Geometry check sheet. Reference: the model listing, model coordinates, mm. Face numbers are marked on the shaded views. A direction names the side the tool comes from. Coordinates: 2 decimals unless noted, no trailing zeros. Order: outer loops, then holes, each group sorted by start corner. A loop starts at its lowest first (then second) coordinate and runs counter-clockwise, first axis right, second up. Notation, with made-up numbers: M 79.25,8 L 93.25,8 A4 cw 93.25,14 Z; hole C 62.5,66 d6. An arc over 180 degrees is marked long. One line per item, written item: value. Start each with the question number.
1) Draft check along X on the marked faces 1, 2 and 3. Enter one of: pulls with the +X half, pulls with the -X half, needs draft (parallel to the pull), parting line crosses it, or undercut.
2) Sectioned sample at A-A, the plane x = 0. Enter the section's corners in (y, z), then the cut area to 3 significant figures.
3) Access from +Z, -Z, +X, -X, +Y, -Y to the whole of each face (thin tool, end or side, straight path). Record for the marked faces 4, 5 and 6.
4) Go/stop test with flat-tipped pins: P1, Ø2, axis at x = -2.5, z = -2, coming from the -Y side; P2, Ø1, axis at x = 0, z = 1, coming from the -Y side; P3, Ø0.5, axis at x = 0, z = -1, coming from the +Y side. Record where each tip stops, or that it passes through.
5) Thickness scan on L1, parallel to Z at x = -3.5, y = -3.5; L2, parallel to X at y = -1, z = -0.8; L3, parallel to Y at x = 0.25, z = -1.65. Record the ranges inside material, lowest first. Write a range as from..to.
```python
from build123d import *

# Parameters (mm, degrees)
SKETCH2_R           = 4.5
BOSS_EXTRUDE1_DEPTH = 3
CUT_EXTRUDE1_DEPTH  = 11.464224768
FILLET1_R           = 0.25


with BuildPart() as part:
    # Sketch1 → Revolve1 (revolve)
    with BuildSketch(Plane(origin=(0, 0, 0), x_dir=(1, 0, 0), z_dir=(0, 1, 0))):
        Polygon((6.5, 0), (0, 0), (0, -2), (6.395184442, -2), align=None)
    revolve(axis=Axis((0, 0, 0), (0, 0, 1)))

    # Sketch2 → Boss-Extrude1 (add)
    with BuildSketch(Plane(origin=(0, 0, 0), x_dir=(-1, 0, 0), z_dir=(0, 0, -1))):
        with Locations(Location((0, 0, 0), (0, 0, 90))):
            Circle(SKETCH2_R)
    extrude(amount=BOSS_EXTRUDE1_DEPTH)

    # Sketch3 → Cut-Extrude1 (cut, through all)
    with BuildSketch(Plane.XY.offset(2)):
        with BuildLine():
            Line((1.568375673, 2.283493649), (1.443375673, 2.5))
            Line((1.443375673, 2.5), (1.193375673, 2.5))
            ThreePointArc((1.193375673, 2.5), (1.043375673, 2.445), (0.893375673, 2.5))
            Line((0.893375673, 2.5), (-0.893375673, 2.5))
            ThreePointArc((-0.893375673, 2.5), (-1.043375673, 2.445), (-1.193375673, 2.5))
            Line((-1.193375673, 2.5), (-1.443375673, 2.5))
            Line((-1.443375673, 2.5), (-1.568375673, 2.283493649))
            ThreePointArc((-1.568375673, 2.283493649), (-1.595744276, 2.126089838), (-1.718375673, 2.023686028))
            Line((-1.718375673, 2.023686028), (-2.611751346, 0.476313972))
            ThreePointArc((-2.611751346, 0.476313972), (-2.639119949, 0.318910162), (-2.761751346, 0.216506351))
            Line((-2.761751346, 0.216506351), (-2.886751346, 0))
            Line((-2.886751346, 0), (-2.761751346, -0.216506351))
            ThreePointArc((-2.761751346, -0.216506351), (-2.639119949, -0.318910162), (-2.611751346, -0.476313972))
            Line((-2.611751346, -0.476313972), (-1.718375673, -2.023686028))
            ThreePointArc((-1.718375673, -2.023686028), (-1.595744276, -2.126089838), (-1.568375673, -2.283493649))
            Line((-1.568375673, -2.283493649), (-1.443375673, -2.5))
            Line((-1.443375673, -2.5), (-1.193375673, -2.5))
            ThreePointArc((-1.193375673, -2.5), (-1.043375673, -2.445), (-0.893375673, -2.5))
            Line((-0.893375673, -2.5), (0.893375673, -2.5))
            ThreePointArc((0.893375673, -2.5), (1.043375673, -2.445), (1.193375673, -2.5))
            Line((1.193375673, -2.5), (1.443375673, -2.5))
            Line((1.443375673, -2.5), (1.568375673, -2.283493649))
            ThreePointArc((1.568375673, -2.283493649), (1.595744276, -2.126089838), (1.718375673, -2.023686028))
            Line((1.718375673, -2.023686028), (2.611751346, -0.476313972))
            ThreePointArc((2.611751346, -0.476313972), (2.639119949, -0.318910162), (2.761751346, -0.216506351))
            Line((2.761751346, -0.216506351), (2.886751346, 0))
            Line((2.886751346, 0), (2.761751346, 0.216506351))
            ThreePointArc((2.761751346, 0.216506351), (2.639119949, 0.318910162), (2.611751346, 0.476313972))
            Line((2.611751346, 0.476313972), (1.718375673, 2.023686028))
            ThreePointArc((1.718375673, 2.023686028), (1.595744276, 2.126089838), (1.568375673, 2.283493649))
        make_face()
    extrude(amount=-CUT_EXTRUDE1_DEPTH, mode=Mode.SUBTRACT)

    # Fillet1
    fillet1_edges = [part.edges().sort_by_distance(p)[0] for p in [
        (-6.395184442, 0, 2),
        (0, -4.5, -3),
    ]]
    fillet(fillet1_edges, radius=FILLET1_R)


solid = part.part
```
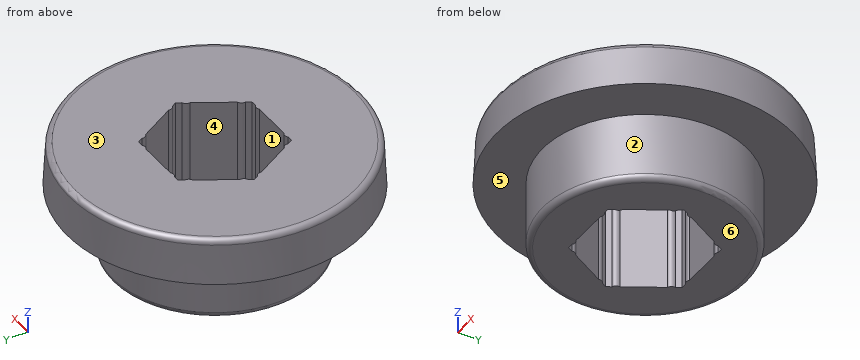
Final values:
1. face 1: undercut
1. face 2: parting line crosses it
1. face 3: needs draft
2. outline: M -6.5,0 L -4.5,0 L -4.5,-2.75 A0.25 ccw -4.25,-3 L -2.5,-3 L -2.5,2 L -6.16,2 A0.25 ccw -6.41,1.76 Z; M 2.5,-3 L 4.25,-3 A0.25 ccw 4.5,-2.75 L 4.5,0 L 6.5,0 L 6.41,1.76 A0.25 ccw 6.16,2 L 2.5,2 Z
2. area: 27.7 mm^2
3. face 4: +Z, -Z
3. face 5: -Z
3. face 6: -Z, +X, -X, +Y, -Y
4. P1: stops at y = -4.24
4. P2: stops at y = -6.47
4. P3: stops at y = 4.5
5. L1: z = 0..2
5. L2: x = -4.39..-2.31, 2.31..4.39
5. L3: y = -4.49..-2.5, 2.5..4.49
